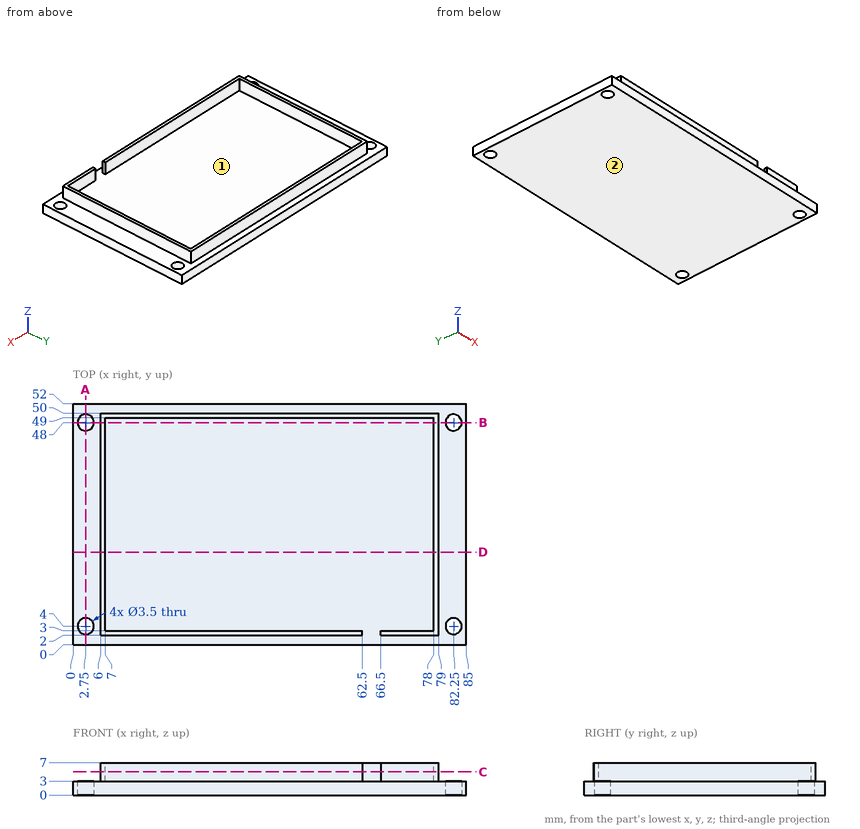
The drawing under review shows one solid part. Ordinate dimensions are in mm from its lowest x, y, z. Round coordinates to 2 decimals unless told otherwise and drop trailing zeros. Order: outer loops, then holes, each group sorted by start corner. A loop starts at its lowest first (then second) coordinate and runs counter-clockwise, first axis right, second up. Notation, with made-up numbers: (26.5, 62.25) -> (47.5, 62.25) arc R20 cw to (47.5, 99.25) -> close; hole circle Ø6 at (-15, -26). An arc over 180 degrees is marked (long way). Use a Markdown table: item, result.
Q1. For line 1 (Y direction, x = 2.75, z = 1.6); line 2 (Y direction, x = 21, z = 5); line 3 (X direction, y = 26, z = 6.5), list the stretches that pass through material, from the lowest coordinate up.
Values:
| item | result |
|---|---|
| line 1 | y = 0 to 2.25, 5.75 to 46.25, 49.75 to 52 |
| line 2 | y = 2 to 3, 49 to 50 |
| line 3 | x = 6 to 7, 78 to 79 |
Q2. Clearance check with flat-ended pins moving along their axes: P1, Ø3, axis at y = 15, z = 5, coming from the -X side; P2, Ø3, axis at x = 60.5, z = 6, coming from the +Y side; P3, Ø1.2, axis at x = 58.5, z = 5.5, coming from the -Y side. State where each tip first meets the part, or that it passes through.
Values:
| item | result |
|---|---|
| P1 | stops at x = 6 |
| P2 | stops at y = 50 |
| P3 | stops at y = 2 |
Q3. Mouldability with a two-part tool opening along X and no side actions: class the marked faces 1 and 2 as +X half, -X half, draft (parallel to the pull), parting line (faces both ways), or undercut.
Values:
| item | result |
|---|---|
| face 1 | undercut |
| face 2 | draft |
Q4. We need section C-C on z = 5. Write out the cut boundary in (x, y), then the cut area to 3 significant figures.
Values:
| item | result |
|---|---|
| outline | (6, 2) -> (62.5, 2) -> (62.5, 3) -> (7, 3) -> (7, 49) -> (78, 49) -> (78, 3) -> (66.5, 3) -> (66.5, 2) -> (79, 2) -> (79, 50) -> (6, 50) -> close |
| area | 234 mm^2 |
Q5. We need section B-B on y = 48. Write out the cut boundary in (x, z).
Values:
| item | result |
|---|---|
| outline | (0, 0) -> (1, 0) -> (1, 3) -> (0, 3) -> close; (4.5, 0) -> (80.5, 0) -> (80.5, 3) -> (79, 3) -> (79, 7) -> (78, 7) -> (78, 3) -> (7, 3) -> (7, 7) -> (6, 7) -> (6, 3) -> (4.5, 3) -> close; (84, 0) -> (85, 0) -> (85, 3) -> (84, 3) -> close |
Q6. We need section A-A on x = 2.75. Write out the cut boundary in (y, z).
Values:
| item | result |
|---|---|
| outline | (0, 0) -> (2.25, 0) -> (2.25, 3) -> (0, 3) -> close; (5.75, 0) -> (46.25, 0) -> (46.25, 3) -> (5.75, 3) -> close; (49.75, 0) -> (52, 0) -> (52, 3) -> (49.75, 3) -> close |
Q7. We need section D-D on y = 20. Write out the cut boundary in (x, z), then the cut area to 3 significant figures.
Values:
| item | result |
|---|---|
| outline | (0, 0) -> (85, 0) -> (85, 3) -> (79, 3) -> (79, 7) -> (78, 7) -> (78, 3) -> (7, 3) -> (7, 7) -> (6, 7) -> (6, 3) -> (0, 3) -> close |
| area | 263 mm^2 |
